Can you work these out from the drawing? Everything is in mm from the part's minimum corner. Coordinates: 2 decimals unless noted, no trailing zeros. Loops run counter-clockwise (first coordinate to the right, second up) from the corner with the lowest first, then second, coordinate; pieces in that order, holes last. Notation, with made-up numbers: M 17.25,12 L 39.25,12 A18 ccw 39.25,16 Z; hole C -22,56 d5. An arc over 180 degrees is marked long. Use CSV: the item, a comma, the result in double quotes. Start each with the question number.
Q1. If we section it at D-D (x = 5): Please give me the cut outline in (y, z), and give its area (3 significant figures).
Q2. If we section it at B-B (y = 5.7): Please give me the cut outline in (x, z).
Q3. Please list where these lines run through material, in increasing order: probe 1 along Z at (x, y) = (2, 5.5); probe 2 along Y at (x, z) = (7, 55.6); probe 3 along Y at (x, z) = (5, 3.2). Write a range as [from, to].
Q4. If we section it at A-A (z = 12): Please give me the cut outline in (x, y).
Q5. If we section it at C-C (x = 8.25): Please give me the cut outline in (y, z), and give its area (3 significant figures).
Q6. For pin 1 Ø1.2 at (x, y) = (5.5, 5) entering from -Z, with a flat end and sliding along its axis, tell me the tip position at first contact or that it passes through.
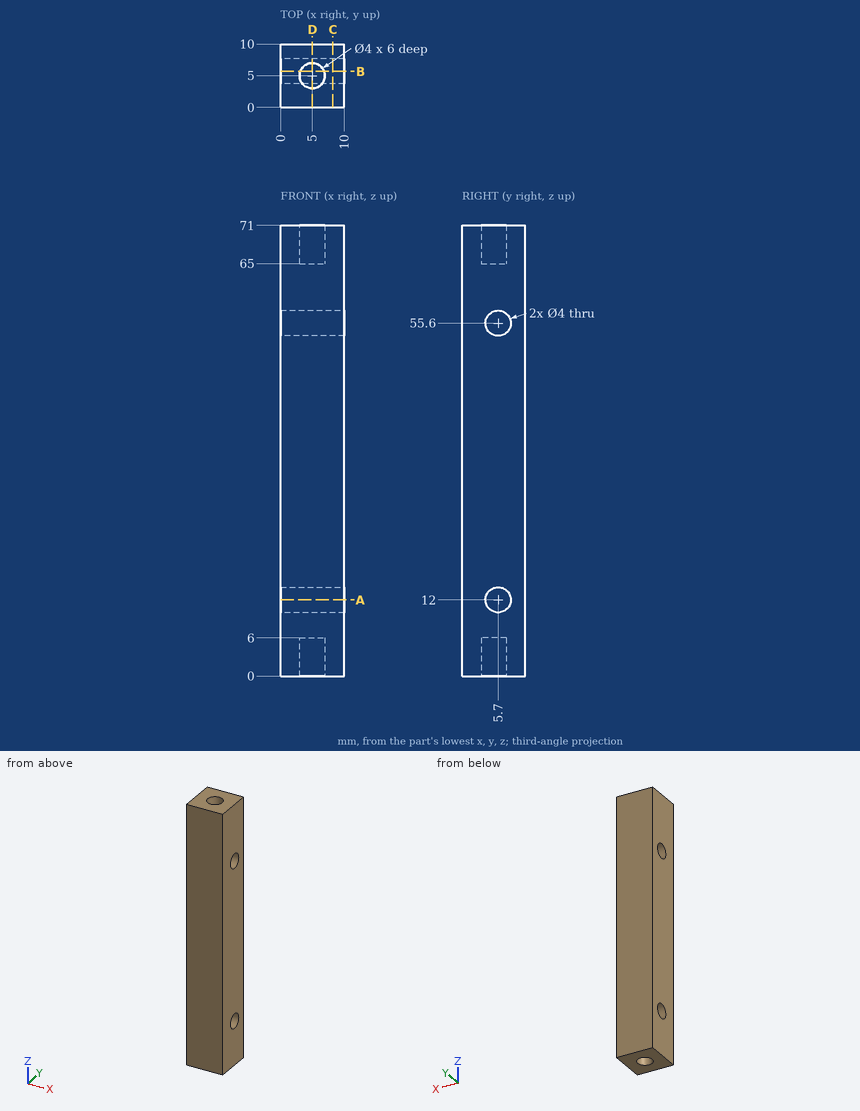
Results below:
1,outline,"M 0,0 L 3,0 L 3,6 L 7,6 L 7,0 L 10,0 L 10,71 L 7,71 L 7,65 L 3,65 L 3,71 L 0,71 Z; hole C 5.7,12 d4; hole C 5.7,55.6 d4"
1,area,"637 mm^2"
2,outline,"M 0,0 L 3.13,0 L 3.13,6 L 6.87,6 L 6.87,0 L 10,0 L 10,10 L 0,10 Z; M 0,14 L 10,14 L 10,53.6 L 0,53.6 Z; M 0,57.6 L 10,57.6 L 10,71 L 6.87,71 L 6.87,65 L 3.13,65 L 3.13,71 L 0,71 Z"
3,probe 1,"[0, 10.01], [13.99, 53.61], [57.59, 71]"
3,probe 2,"[0, 3.7], [7.7, 10]"
3,probe 3,"[0, 3], [7, 10]"
4,outline,"M 0,0 L 10,0 L 10,3.7 L 0,3.7 Z; M 0,7.7 L 10,7.7 L 10,10 L 0,10 Z"
5,outline,"M 0,0 L 10,0 L 10,71 L 0,71 Z; hole C 5.7,12 d4; hole C 5.7,55.6 d4"
5,area,"685 mm^2"
6,pin 1,"z = 6"
